```python
from build123d import *

# Parameters (mm, degrees)
BOSS_EXTRUDE1_DEPTH = 3


with BuildPart() as part:
    # Sketch1 → Boss-Extrude1 (new body)
    with BuildSketch(Plane(origin=(0, 0, 0), x_dir=(1, 0, 0), z_dir=(0, 1, 0))):
        with BuildLine():
            Line((0, 0), (3.8, 0))
            Line((3.8, 0), (3.8, -5.815800771))
            ThreePointArc((3.8, -5.815800771), (3.475312858, -6.553332156), (2.712094913, -6.811929626))
            Line((2.712094913, -6.811929626), (-5.163624241, -6.116923376))
            ThreePointArc((-5.163624241, -6.116923376), (-6.238909118, -5.813137084), (-7.128441398, -5.136930013))
            ThreePointArc((-7.128441398, -5.136930013), (-9.7, 1.557713995), (-7.128441398, 8.252358003))
            ThreePointArc((-7.128441398, 8.252358003), (-6.219292824, 8.938259935), (-5.120004532, 9.235880232))
            Line((-5.120004532, 9.235880232), (2.726634816, 9.813105915))
            ThreePointArc((2.726634816, 9.813105915), (3.48067423, 9.548387007), (3.8, 8.815800771))
            Line((3.8, 8.815800771), (3.8, 3))
            Line((3.8, 3), (0, 3))
            ThreePointArc((0, 3), (-1.5, 1.5), (0, 0))
        make_face()
    extrude(amount=BOSS_EXTRUDE1_DEPTH)


solid = part.part
```
Work out the finished part from the listing and answer in its coordinate system (mm). A direction names the side the tool comes from. Coordinates: 2 decimals unless noted, no trailing zeros. Write each loop counter-clockwise with the first axis right and the second up, starting at its lowest first coordinate (ties: lowest second). Pieces come first, ordered by that corner, then holes. Notation, with made-up numbers: (21, 83.5) - (52, 83.5) arc R18 ccw to (52, 87.5) - close; hole circle Ø9 at (15.5, -25). An arc over 180 degrees is marked (long way). Answer as a JSON object with one key per item and string values.
Q1. Given pin 1 Ø1.5 at (x, y) = (1, 1) entering from -Z; pin 2 Ø1 at (y, z) = (1, -6.5) entering from -X; pin 3 Ø1 at (x, y) = (-0.5, 2) entering from +Z, each flat-ended and moving along its own axis, determine where each tip first touches the part or whether it passes through.
Results list:
{"pin 1": "stops at z = -9.74", "pin 2": "stops at x = -8.66", "pin 3": "stops at z = 6.57"}
Q2. Find section A-A (x = -1). Write down the section's boundary in (y, z).
Results list:
{"outline": "(0, -9.54) - (3, -9.54) - (3, -2.62) - (0, -2.62) - close; (0, -0.38) - (3, -0.38) - (3, 6.48) - (0, 6.48) - close"}
Q3. Find section C-C (z = 3.75). Write down the section's boundary in (x, y), plus the area to 3 significant figures.
Results list:
{"outline": "(-8.18, 0) - (3.8, 0) - (3.8, 3) - (-8.18, 3) - close", "area": "35.9 mm^2"}
Q4. Find section D-D (x = -5.75). Write down the section's boundary in (y, z), plus the area to 3 significant figures.
Results list:
{"outline": "(0, -9.12) - (3, -9.12) - (3, 6.01) - (0, 6.01) - close", "area": "45.4 mm^2"}
Q5. Which of the six approach directions +Z, -Z, +X, -X, +Y, -Y give full straight-line access (tool end or side, diameter ignored) to faces 1 (the flat face through (-3, 3, -2)), 2 (the flat face through (2, 1, 0))?
Results list:
{"face 1": "+Z, -Z, +X, -X, +Y", "face 2": "+X, +Y, -Y"}
Q6. Consider L1, parallel to Z at x = 0.5, y = 1.1; L2, parallel to Z at x = 1.25, y = 1.3; L3, parallel to X at y = 2.85, z = 4.5. Determine where each line is inside the solid, lowest interval first. Write a range as from..to.
Results list:
{"L1": "z = -9.65..-3, 0..6.62", "L2": "z = -9.7..-3, 0..6.68", "L3": "x = -7.66..3.8"}
Q7. Find section B-B (y = 2.35). Write down the section's boundary in (x, z), plus the area to 3 significant figures.
Results list:
{"outline": "(-7.13, -8.25) arc R3 ccw to (-5.12, -9.24) - (2.73, -9.81) arc R1 ccw to (3.8, -8.82) - (3.8, -3) - (0, -3) arc R1.5 cw to (0, 0) - (3.8, 0) - (3.8, 5.82) arc R1 ccw to (2.71, 6.81) - (-5.16, 6.12) arc R3 ccw to (-7.13, 5.14) arc R10 ccw to start", "area": "181 mm^2"}
Q8. For a pull along Z with two mould halves and no side action, classify faces 3 (the cylindrical face through (-6.234, 1.479, -8.931)), 4 (the flat face through (2, 1, -3)), 5 (the flat face through (3.8, 1, 3)), 6 (the cylindrical face through (-9.7, 1.5, -1.5)) as pulls with the +Z half, pulls with the -Z half, needs draft (parallel to the pull), parting line crosses it, or undercut.
Results list:
{"face 3": "pulls with the -Z half", "face 4": "undercut", "face 5": "needs draft", "face 6": "parting line crosses it"}
